Print and shaded views of the part. All mm, measured from the part's lowest x, y and z. Round coordinates to 2 decimals unless told otherwise and drop trailing zeros. Write each loop counter-clockwise with the first axis right and the second up, starting at its lowest first coordinate (ties: lowest second). Pieces come first, ordered by that corner, then holes. Notation, with made-up numbers: (-38.5, -8.75) -> (-23.5, -8.75) arc R24 ccw to (-23.5, 8.25) -> close; hole circle Ø5 at (52.25, 34.25). An arc over 180 degrees is marked (long way). Return JSON: item names as keys, results as strings. Group by question number.
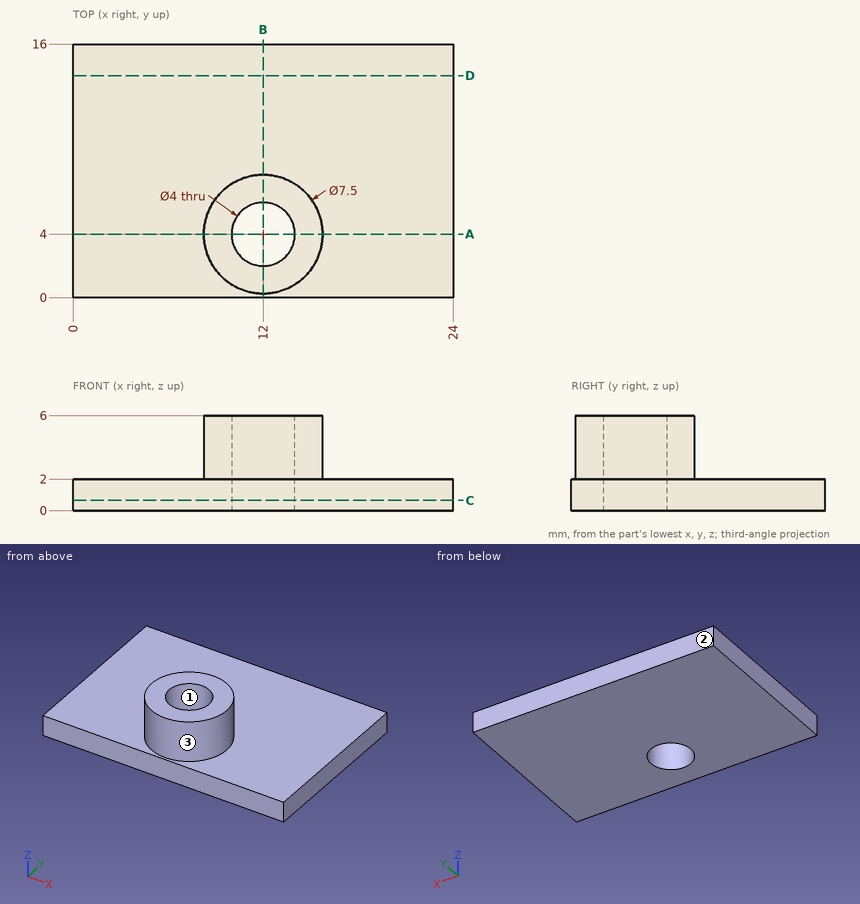
Item 1: Cut at A-A (y = 4). Write the cut outline in (x, z), then the cut area to 3 significant figures.
Item 2: Wall check: L1, parallel to Y at x = 12, z = 2.15; L2, parallel to Y at x = 12, z = 1.4; L3, parallel to Z at x = 16.75, y = 3.25. Give the ranges that are in metal, low to high.
Item 3: Cut at D-D (y = 14). Write the cut outline in (x, z), then the cut area to 3 significant figures.
Item 4: Flat gauge pin, fed straight in: P1, Ø2.5, axis at x = 12, y = 4, coming from the +Z side. Where does the tip first touch, or does it go through?
Item 5: Two-plate mould, pull along X, no slides. Class the marked faces 1, 2 and 3: released by +X, released by -X, zero draft, split by the parting line, or undercut.
Item 6: Cut at C-C (z = 0.65). Write the cut outline in (x, y).
Item 7: Cut at B-B (x = 12). Write the cut outline in (y, z), then the cut area to 3 significant figures.
Checks:
{
 "1": {"outline": "(0, 0) -> (10, 0) -> (10, 6) -> (8.25, 6) -> (8.25, 2) -> (0, 2) -> close; (14, 0) -> (24, 0) -> (24, 2) -> (15.75, 2) -> (15.75, 6) -> (14, 6) -> close", "area": "54.0 mm2"},
 "2": {"L1": "y = 0.25 to 2, 6 to 7.75", "L2": "y = 0 to 2, 6 to 16", "L3": "z = 0 to 2"},
 "3": {"outline": "(0, 0) -> (24, 0) -> (24, 2) -> (0, 2) -> close", "area": "48.0 mm2"},
 "4": {"P1": "passes through"},
 "5": {"face 1": "undercut", "face 2": "zero draft", "face 3": "split by the parting line"},
 "6": {"outline": "(0, 0) -> (24, 0) -> (24, 16) -> (0, 16) -> close; hole circle Ø4 at (12, 4)"},
 "7": {"outline": "(0, 0) -> (2, 0) -> (2, 6) -> (0.25, 6) -> (0.25, 2) -> (0, 2) -> close; (6, 0) -> (16, 0) -> (16, 2) -> (7.75, 2) -> (7.75, 6) -> (6, 6) -> close", "area": "38.0 mm2"}
}
